The listing builds one solid part. Answer for the finished solid, in the listing's coordinates (mm). Face numbers are marked on the shaded views. A direction names the side the tool comes from. Give positions to 0.01 mm unless a question says otherwise; leave off trailing zeros. Write each loop counter-clockwise with the first axis right and the second up, starting at its lowest first coordinate (ties: lowest second). Pieces come first, ordered by that corner, then holes. Notation, with made-up numbers: (13, 57.5) - (72, 57.5) arc R13 cw to (72, 80.5) - close; hole circle Ø1 at (-31, 27.25). An arc over 180 degrees is marked (long way). Answer in a Markdown table with one row per item. Add a question column.
from build123d import *

# Parameters (mm, degrees)
BOSS_EXTRUDE1_DEPTH = 11.7602
FILLET2_R           = 2.54
FILLET3_R           = 2.54
SKETCH3_R           = 1.55
CUT_EXTRUDE1_DEPTH  = 1.524


with BuildPart() as part:
    # Sketch2 → Boss-Extrude1 (new body)
    with BuildSketch(Plane.XY):
        Polygon((0, 0), (7.62, 0), (7.62, 9.9949), (19.6596, 9.9949), (19.6596, 0), (27.2796, 0), (27.2796, 1.524), (21.1836, 1.524), (21.1836, 11.5189), (6.096, 11.5189), (6.096, 1.524), (0, 1.524), align=None)
    extrude(amount=BOSS_EXTRUDE1_DEPTH)

    # Fillet2
    fillet2_edges = [part.edges().sort_by_distance(p)[0] for p in [
        (21.1836, 11.5189, 5.8801),
    ]]
    fillet(fillet2_edges, radius=FILLET2_R)

    # Fillet3
    fillet3_edges = [part.edges().sort_by_distance(p)[0] for p in [
        (6.096, 11.5189, 5.8801),
    ]]
    fillet(fillet3_edges, radius=FILLET3_R)

    # Sketch3 → Cut-Extrude1 (cut)
    with BuildSketch(Plane(origin=(0, 0, 0), x_dir=(1, 0, 0), z_dir=(0, 1, 0))):
        with Locations((3.048, -5.8801)):
            Circle(SKETCH3_R)
        with Locations((24.2316, -5.8801)):
            Circle(SKETCH3_R)
    extrude(amount=CUT_EXTRUDE1_DEPTH, mode=Mode.SUBTRACT)


solid = part.part
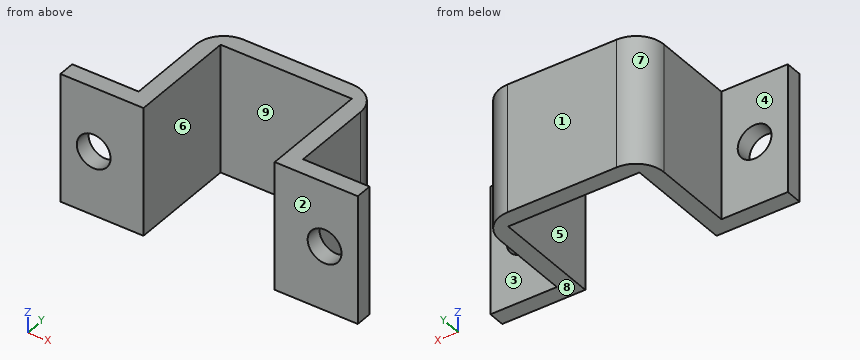
1. Straight lines are drawn through the part: L1, parallel to X at y = 7.75, z = 8; L2, parallel to X at y = 1, z = 5; L3, parallel to X at y = 0.75, z = 3.5. For each, find the intervals that lie inside material, in ascending order. Write a range as [from, to].
2. The mould has two halves that part along X. Classify the marked faces 6, 7, 8 and 9: +X half, -X half, draft (parallel to the pull), parting line (faces both ways), or undercut.
3. Section A-A (y = 4.25) is taken. Give the vertices of the cut face in (x, z).
4. Section B-B (z = 5.5) is taken. Give the vertices of the cut face in (x, y).
5. Given pin 1 Ø1.5 at (x, y) = (5, 10.5) entering from -Z; pin 2 Ø3 at (x, z) = (3.5, 8) entering from +Y; pin 3 Ø6 at (x, z) = (16.5, 5.5) entering from -Y; pin 4 Ø2 at (y, z) = (5, 9) entering from -X, each flat-ended and moving along its own axis, determine where each tip first touches the part or whether it passes through.
6. Section C-C (y = 1) is taken. Give the vertices of the cut face in (x, z), and give its area (3 significant figures).
7. A tool of negligible diameter and unlimited length cuts with its end or side. For the marked faces 1, 2, 3, 4 and 5, from which of +Z, -Z, +X, -X, +Y, -Y can it reach the whole face along a straight path? Write none if from no direction.
8. Section D-D (z = 1.75) is taken. Give the vertices of the cut face in (x, y).
Geometry check:
| question | item | result |
|---|---|---|
| 1 | L1 | [6.1, 7.62], [19.66, 21.18] |
| 1 | L2 | [0, 1.77], [4.32, 7.62], [19.66, 22.96], [25.51, 27.28] |
| 1 | L3 | [0, 7.62], [19.66, 27.28] |
| 2 | face 6 | undercut |
| 2 | face 7 | -X half |
| 2 | face 8 | draft |
| 2 | face 9 | undercut |
| 3 | outline | (6.1, 0) - (7.62, 0) - (7.62, 11.76) - (6.1, 11.76) - close; (19.66, 0) - (21.18, 0) - (21.18, 11.76) - (19.66, 11.76) - close |
| 4 | outline | (0, 0) - (1.55, 0) - (1.55, 1.52) - (0, 1.52) - close; (4.55, 0) - (7.62, 0) - (7.62, 9.99) - (19.66, 9.99) - (19.66, 0) - (22.73, 0) - (22.73, 1.52) - (21.18, 1.52) - (21.18, 8.98) arc R2.54 ccw to (18.64, 11.52) - (8.64, 11.52) arc R2.54 ccw to (6.1, 8.98) - (6.1, 1.52) - (4.55, 1.52) - close; (25.73, 0) - (27.28, 0) - (27.28, 1.52) - (25.73, 1.52) - close |
| 5 | pin 1 | through |
| 5 | pin 2 | y = 1.52 |
| 5 | pin 3 | y = 9.99 |
| 5 | pin 4 | x = 6.1 |
| 6 | outline | (0, 0) - (7.62, 0) - (7.62, 11.76) - (0, 11.76) - close; (19.66, 0) - (27.28, 0) - (27.28, 11.76) - (19.66, 11.76) - close; hole circle Ø3.1 at (3.05, 5.88); hole circle Ø3.1 at (24.23, 5.88) |
| 6 | area | 164 mm² |
| 7 | face 1 | +Z, -Z, +X, -X, +Y |
| 7 | face 2 | +Z, -Z, +X, -X, -Y |
| 7 | face 3 | +Z, -Z, +X, +Y |
| 7 | face 4 | +Z, -Z, -X, +Y |
| 7 | face 5 | +Z, -Z, -Y |
| 8 | outline | (0, 0) - (7.62, 0) - (7.62, 9.99) - (19.66, 9.99) - (19.66, 0) - (27.28, 0) - (27.28, 1.52) - (21.18, 1.52) - (21.18, 8.98) arc R2.54 ccw to (18.64, 11.52) - (8.64, 11.52) arc R2.54 ccw to (6.1, 8.98) - (6.1, 1.52) - (0, 1.52) - close |
